Can you work these out from the model? Positions are in its coordinate system, mm. A direction names the side the tool comes from. Give positions to 0.01 mm unless a question says otherwise; leave off trailing zeros. Order: outer loops, then holes, each group sorted by start corner. A loop starts at its lowest first (then second) coordinate and runs counter-clockwise, first axis right, second up. Notation, with made-up numbers: (53.5, 1.25) -> (61.5, 1.25) arc R16 cw to (61.5, 26.25) -> close; hole circle Ø10 at (-6.75, -25.75). An arc over 180 degrees is marked (long way). Answer as a JSON object with one key per item and string values.
```python
from build123d import *

# Parameters (mm, degrees)
F1_DEPTH = 89


with BuildPart() as f1:
    # F0 (on Top) → F1 (new body)
    with BuildSketch(Plane.XY):
        with BuildLine():
            ThreePointArc((-2, 47.4578760587), (-32.8728611472, -34.287388352), (47.5, 0))
            ThreePointArc((47.5, 0), (34.287388352, 32.8728611472), (2, 47.4578760587))
            Line((2, 47.4578760587), (2, 34.9655821919))
            Line((2, 34.9655821919), (0, 34.9655821919))
            Line((0, 34.9655821919), (-2, 34.9655821919))
            Line((-2, 34.9655821919), (-2, 47.4578760587))
        make_face()
    extrude(amount=F1_DEPTH)


solid = f1.part
```
1. For faces 4 (the face through (-1, 1, 89)), 5 (the face through (2, 41, 44)), which set-ups out of +Z, -Z, +X, -X, +Y, -Y let a thin tool reach every point of the face, with its end or its side?
Worked answers:
{"face 4": "+Z, +X, -X, +Y, -Y", "face 5": "+Z, -Z, +Y"}
2. Please list where these lines run through material, in increasing order: L1, parallel to X at y = 36.5, z = 58; L2, parallel to Y at x = -39.5, z = 54.5; L3, parallel to Y at x = -16, z = 28.
Worked answers:
{"L1": "-30.4 to -2, 2 to 30.4", "L2": "-26.38 to 26.38", "L3": "-44.72 to 44.72"}
3. If we section it at A-A on z = 63: Please give me the cut outline in (x, y).
Worked answers:
{"outline": "(-2, 34.97) -> (-2, 47.46) arc R47.5 ccw (long way) to (2, 47.46) -> (2, 34.97) -> close"}
4. If we mould it in two halves opening along X, with no side actions, what happens to faces 1 (the face through (0, 34.966, 44)), 2 (the face through (-1, 1, 0)), 3 (the face through (-2, 41, 44))? For each: +X half, -X half, draft (parallel to the pull), parting line (faces both ways), or undercut.
Worked answers:
{"face 1": "undercut", "face 2": "draft", "face 3": "undercut"}
5. Will these pins go through, and if not, where does the flat tip stop? pin 1 Ø10 at (y, z) = (18.5, 54) entering from +X; pin 2 Ø1.5 at (x, z) = (-28.5, 18.5) entering from -Y; pin 3 Ø1.2 at (x, z) = (0.5, 42) entering from +Y.
Worked answers:
{"pin 1": "x = 45.54", "pin 2": "y = -38.55", "pin 3": "y = 34.97"}
6. If we section it at C-C on y = -23: Please give me the cut outline in (x, z).
Worked answers:
{"outline": "(-41.56, 0) -> (41.56, 0) -> (41.56, 89) -> (-41.56, 89) -> close"}
7. If we section it at B-B on x = 0: Please give me the cut outline in (y, z).
Worked answers:
{"outline": "(-47.5, 0) -> (34.97, 0) -> (34.97, 89) -> (-47.5, 89) -> close"}
